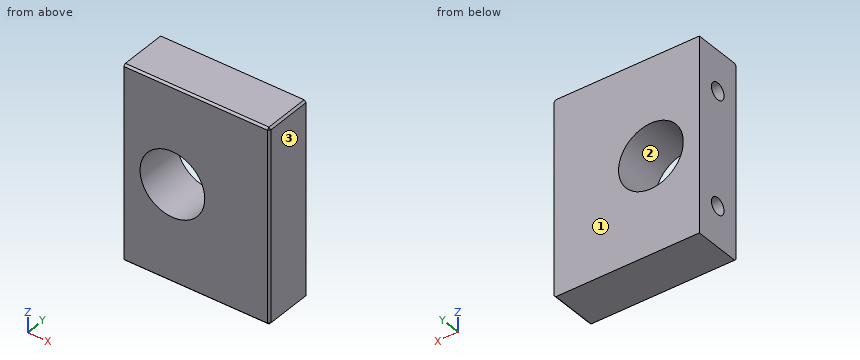
from build123d import *

# Parameters (mm, degrees)
F0_W     = 57.15
F0_H     = 76.2
F0_R     = 12.7127
F1_DEPTH = 19.05
F3_D     = 6.5278
F3_DEPTH = 16.002
F3_TIP   = 1.9611489744
F4_SIZE2 = 0.762
F4_SIZE  = 0.762


with BuildPart() as f1:
    # F0 (on Front) → F1 (new body)
    with BuildSketch(Plane.XZ):
        with Locations((28.575, 38.1)):
            Rectangle(F0_W, F0_H)
        with Locations((19.05, 38.1)):
            Circle(F0_R, mode=Mode.SUBTRACT)
    extrude(amount=F1_DEPTH)

    # F3
    with Locations(Plane(origin=(0, 0, 0), x_dir=(0, -1, 0), z_dir=(-1, 0, 0))):
        with Locations((9.525, 60.325), (9.525, 15.875)):
            Hole(F3_D / 2, depth=F3_DEPTH)
            with Locations((0, 0, -(F3_DEPTH + F3_TIP / 2))):  # 118° drill point
                Cone(0, F3_D / 2, F3_TIP, mode=Mode.SUBTRACT)

    # F4
    f4_edges = [f1.edges().sort_by_distance(p)[0] for p in [
        (57.15, -19.05, 38.1),
        (28.575, -19.05, 76.2),
        (28.575, -19.05, 0),
        (57.15, -9.525, 76.2),
        (57.15, -9.525, 0),
    ]]
    chamfer(f4_edges, length=F4_SIZE, length2=F4_SIZE2)


solid = f1.part
Here's how the part is built. I have some questions about the finished solid (model axes, mm). Face numbers are marked on the shaded views. Round coordinates to 2 decimals unless told otherwise and drop trailing zeros. Write each loop counter-clockwise with the first axis right and the second up, starting at its lowest first coordinate (ties: lowest second). Pieces come first, ordered by that corner, then holes.
1. If we mould it in two halves opening along X, with no side actions, what happens to the marked faces 1, 2 and 3? For each: released by +X, released by -X, zero draft, split by the parting line, or undercut.
2. Suppose I cut it at A-A (z = 38.1). List the corners of the cut face in (x, y) for me.
3. Will these pins go through, and if not, where does the flat tip stop? pin 1 Ø3 at (x, z) = (10.5, 32.5) entering from +Y; pin 2 Ø5 at (y, z) = (-9.525, 60.325) entering from -X.
4. Suppose I cut it at B-B (y = -2). List the corners of the cut face in (x, z) for me.
5. Suppose I cut it at C-C (x = 19.05). List the corners of the cut face in (y, z) for me, and give its area (3 significant figures).
6. I need wall thicknesses on L1, parallel to Z at x = 19.05, y = -4.25; L2, parallel to Z at x = 8, y = -5.5; L3, parallel to X at y = -10, z = 37.5. Which ranges of each line are inside material? Lowest first, please.
7. Suppose I cut it at D-D (x = 9). List the corners of the cut face in (y, z) for me (3 decimals), and give its area (3 significant figures).
Answer sheet:
1. face 1: zero draft
1. face 2: undercut
1. face 3: released by +X
2. outline: (0, -19.05) - (6.34, -19.05) - (6.34, 0) - (0, 0) - close; (31.76, -19.05) - (56.39, -19.05) - (57.15, -18.29) - (57.15, 0) - (31.76, 0) - close
3. pin 1: passes through
3. pin 2: stops at x = 16.46
4. outline: (0, 0) - (56.39, 0) - (57.15, 0.76) - (57.15, 75.44) - (56.39, 76.2) - (0, 76.2) - close; hole circle Ø25.43 at (19.05, 38.1)
5. outline: (-19.05, 0.76) - (-18.29, 0) - (0, 0) - (0, 25.39) - (-19.05, 25.39) - close; (-19.05, 50.81) - (0, 50.81) - (0, 76.2) - (-18.29, 76.2) - (-19.05, 75.44) - close
5. area: 967 mm2
6. L1: z = 0 to 25.39, 50.81 to 76.2
6. L2: z = 0 to 31.81, 44.39 to 76.2
6. L3: x = 0 to 6.35, 31.75 to 57.15
7. outline: (-19.05, 0.762) - (-18.288, 0) - (0, 0) - (0, 30.315) - (-19.05, 30.315) - close; (-19.05, 45.885) - (0, 45.885) - (0, 76.2) - (-18.288, 76.2) - (-19.05, 75.438) - close; hole circle Ø6.528 at (-9.525, 15.875); hole circle Ø6.528 at (-9.525, 60.325)
7. area: 1,090 mm2
